For this review, use the dimensioned drawing (mm, ordinates from the lowest corner) and the shaded views. Round coordinates to 2 decimals unless told otherwise and drop trailing zeros. Order: outer loops, then holes, each group sorted by start corner. A loop starts at its lowest first (then second) coordinate and runs counter-clockwise, first axis right, second up. Notation, with made-up numbers: (9.25, 19) -> (36.25, 19) arc R20 ccw to (36.25, 41) -> close; hole circle Ø4 at (-22.75, -38). An arc over 180 degrees is marked (long way). Answer in a Markdown table with one row per item.
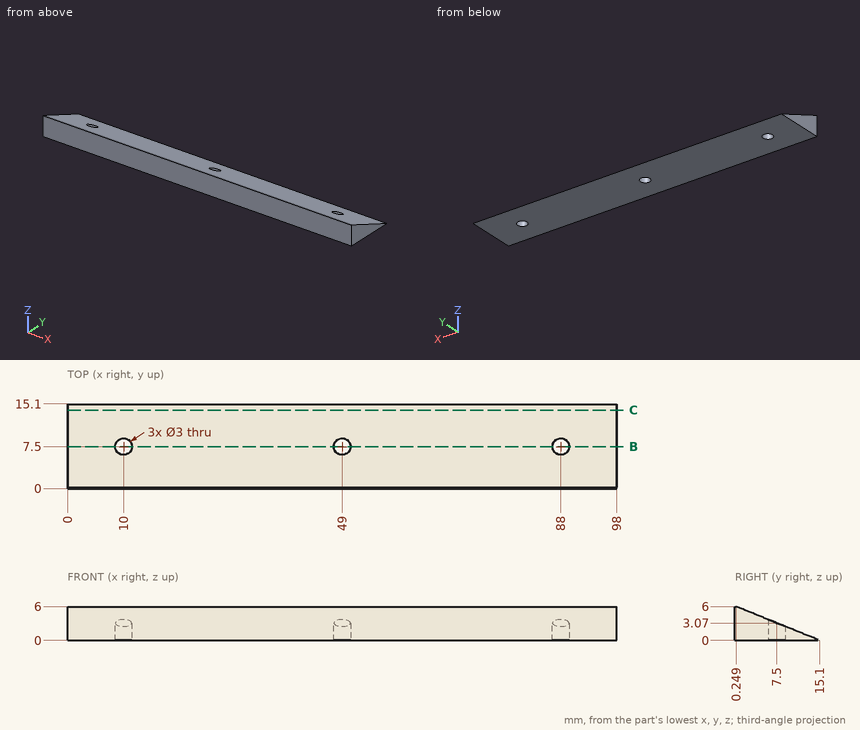
Q1. To check wall thickness, follow probe 1 along X at (y, z) = (7.5, 1.6); probe 2 along Y at (x, z) = (49, 2.9); probe 3 along Z at (x, y) = (41, 6) (1 decimal). State the ranges of each line that lie inside material, in increasing order.
Answer key:
| item | result |
|---|---|
| probe 1 | x = 0 to 8.5, 11.5 to 47.5, 50.5 to 86.5, 89.5 to 98 |
| probe 2 | y = 0 to 6 |
| probe 3 | z = 0 to 3.7 |
Q2. Take a section at C-C, the plane y = 14. Write out the cut boundary in (x, z) (1 decimal).
Answer key:
| item | result |
|---|---|
| outline | (0, 0) -> (98, 0) -> (98, 0.4) -> (0, 0.4) -> close |
Q3. Clearance check with flat-ended pins moving along their axes: pin 1 Ø5 at (x, y) = (10, 7.5) entering from +Z; pin 2 Ø1.5 at (x, y) = (29.5, 12.5) entering from +Z; pin 3 Ø8 at (x, y) = (84, 13) entering from +Z (1 decimal). State where each tip first meets the part, or that it passes through.
Answer key:
| item | result |
|---|---|
| pin 1 | stops at z = 4.08 |
| pin 2 | stops at z = 1.35 |
| pin 3 | stops at z = 2.5 |
Q4. Take a section at B-B, the plane y = 7.5. Write out the cut boundary in (x, z), then the cut area to 3 significant figures.
Answer key:
| item | result |
|---|---|
| outline | (0, 0) -> (8.5, 0) -> (8.5, 3.07) -> (0, 3.07) -> close; (11.5, 0) -> (47.5, 0) -> (47.5, 3.07) -> (11.5, 3.07) -> close; (50.5, 0) -> (86.5, 0) -> (86.5, 3.07) -> (50.5, 3.07) -> close; (89.5, 0) -> (98, 0) -> (98, 3.07) -> (89.5, 3.07) -> close |
| area | 273 mm^2 |
